Model file for the job. Use its own axes, mm. A direction names the side the tool comes from. Round coordinates to 2 decimals unless told otherwise and drop trailing zeros. Order: outer loops, then holes, each group sorted by start corner. A loop starts at its lowest first (then second) coordinate and runs counter-clockwise, first axis right, second up. Notation, with made-up numbers: M -38,82.5 L -26,82.5 A32 cw -26,120.5 Z; hole C 9.5,8 d10. An arc over 180 degrees is marked long. Return JSON: item names as keys, results as strings. Group by question number.
Item 1: Pin check, flat tips, straight feed: pin 1 Ø2 at (y, z) = (67, 20) entering from -X; pin 2 Ø2.5 at (y, z) = (116, 45) entering from -X. Stop position of each tip, or through.
Item 2: Slice it at D-D on y = 101. Write the cut outline in (x, z).
Item 3: Pull direction Z, two halves, no side cores. Call faces 5 (the face through (248.028, 86.113, 33.306)), 6 (the face through (124, 3, 0)), 7 (the face through (123, 4, 30)): pulls with the +Z half, pulls with the -Z half, needs draft (parallel to the pull), parting line crosses it, or undercut.
Item 4: Slice it at C-C on z = 53.5. Write the cut outline in (x, y).
Item 5: Probe line 1 along X through (y, z) = (15.5, 39.5); line 2 along Y through (x, z) = (59, 42); line 3 along X through (y, z) = (94.5, 42). List the from-to ranges inside material, lowest first.
Item 6: Which spindle directions (+Z, -Z, +X, -X, +Y, -Y) get a long thin tool onto all of the face, cutting with end or side? Do faces 1 (the face through (248, 65.3, 35.4)), 2 (the face through (123, 121, 30)), 3 (the face through (1.97, 53.22, 17.9)), 4 (the face through (247.01, 58.7, 33.91)). Say none if no direction does.
Item 7: Slice it at A-A on x = 156. Write the cut outline in (y, z).
Item 8: Slice it at B-B on y = 9. Write the cut outline in (x, z), then the cut area to 3 significant figures.
from build123d import *

# Parameters (mm, degrees)
SKIZZE1_W                       = 250
SKIZZE1_H                       = 125
SKIZZE1_W_2                     = 242
SKIZZE1_H_2                     = 117
AUFSATZ_LINEAR_AUSTRAGEN1_DEPTH = 60
SKIZZE2_R                       = 15.25
SKIZZE2_R_2                     = 2
SCHNITT_LINEAR_AUSTRAGEN1_DEPTH = 10
SKIZZE8_R                       = 15.25
SKIZZE8_R_2                     = 2
SCHNITT_LINEAR_AUSTRAGEN6_DEPTH = 22
SKIZZE10_W                      = 23.41492783
SKIZZE10_H                      = 23.41492783
SCHNITT_LINEAR_AUSTRAGEN7_DEPTH = 2


with BuildPart() as part:
    # Skizze1 → Aufsatz-Linear austragen1 (new body)
    with BuildSketch(Plane.XY):
        with Locations((125, 62.5)):
            Rectangle(SKIZZE1_W, SKIZZE1_H)
        with Locations((125, 62.5)):
            Rectangle(SKIZZE1_W_2, SKIZZE1_H_2, mode=Mode.SUBTRACT)
    extrude(amount=AUFSATZ_LINEAR_AUSTRAGEN1_DEPTH)

    # Skizze2 → Schnitt-Linear austragen1 (cut)
    with BuildSketch(Plane.ZY):
        with Locations((30, 62.5)):
            Circle(SKIZZE2_R)
        with Locations((15, 77.5)):
            Circle(SKIZZE2_R_2)
        with Locations((45, 77.5)):
            Circle(SKIZZE2_R_2)
        with Locations((45, 47.5)):
            Circle(SKIZZE2_R_2)
        with Locations((15, 47.5)):
            Circle(SKIZZE2_R_2)
    extrude(amount=-SCHNITT_LINEAR_AUSTRAGEN1_DEPTH, mode=Mode.SUBTRACT)

    # Skizze8 → Schnitt-Linear austragen6 (cut)
    with BuildSketch(Plane(origin=(250, 0, 0), x_dir=(0, 0, -1), z_dir=(1, 0, 0))):
        with Locations((-30, 101)):
            Circle(SKIZZE8_R)
        with Locations((-45, 116)):
            Circle(SKIZZE8_R_2)
        with Locations((-15, 86)):
            Circle(SKIZZE8_R_2)
        with Locations((-45, 86)):
            Circle(SKIZZE8_R_2)
        with Locations((-15, 116)):
            Circle(SKIZZE8_R_2)
        Polygon((-30, 70.207463915), (-37.707463915, 62.5), (-30, 54.792536085), (-22.292536085, 62.5), align=None)
    extrude(amount=-SCHNITT_LINEAR_AUSTRAGEN6_DEPTH, mode=Mode.SUBTRACT)

    # Skizze10 → Schnitt-Linear austragen7 (cut)
    with BuildSketch(Plane(origin=(250, 0, 0), x_dir=(0, 0, -1), z_dir=(1, 0, 0))):
        with Locations((-30, 62.5)):
            Rectangle(SKIZZE10_W, SKIZZE10_H)
    extrude(amount=-SCHNITT_LINEAR_AUSTRAGEN7_DEPTH, mode=Mode.SUBTRACT)


solid = part.part
Output values:
{
 "1": {"pin 1": "x = 246", "pin 2": "x = 0"},
 "2": {"outline": "M 0,0 L 4,0 L 4,60 L 0,60 Z; M 246,0 L 250,0 L 250,14.75 L 246,14.75 Z; M 246,45.25 L 250,45.25 L 250,60 L 246,60 Z"},
 "3": {"face 5": "undercut", "face 6": "pulls with the -Z half", "face 7": "needs draft"},
 "4": {"outline": "M 0,0 L 250,0 L 250,125 L 0,125 Z; hole M 4,4 L 246,4 L 246,121 L 4,121 Z"},
 "5": {"line 1": "0 to 4, 246 to 250", "line 2": "0 to 4, 121 to 125", "line 3": "0 to 4"},
 "6": {"face 1": "+X", "face 2": "+Z, -Z", "face 3": "-X", "face 4": "+X, -X"},
 "7": {"outline": "M 0,0 L 4,0 L 4,60 L 0,60 Z; M 121,0 L 125,0 L 125,60 L 121,60 Z"},
 "8": {"outline": "M 0,0 L 4,0 L 4,60 L 0,60 Z; M 246,0 L 250,0 L 250,60 L 246,60 Z", "area": "480 mm²"}
}
